Input: part model. Units: mm. Frame: model coordinates. A direction names the side the tool comes from. Round coordinates to 2 decimals unless told otherwise and drop trailing zeros. Loops run counter-clockwise (first coordinate to the right, second up) from the corner with the lowest first, then second, coordinate; pieces in that order, holes last. Notation, with made-up numbers: M 63,-7 L 94,-7 A20 cw 94,2 Z; hole C -24.75,-26 d6. An arc over 180 degrees is marked long. Return JSON: item names as keys, results as strings. Group by question number.
1) Access query for faces 5 (the face through (-66.951, 26, -28)), 6 (the face through (-55, 26, -14)), 7 (the face through (36.8, 56.6, 2.5)), 8 (the face through (-14, 54, 5)), 9 (the face through (-76.951, 29, -27)). Directions: +Z, -Z, +X, -X, +Y, -Y. A direction counts if a zero-diameter tool reaches every point of the face in a straight line with its end or side. Return the directions, or none.
2) Material intervals for line 1 (X direction, y = 29.5, z = -5); line 2 (X direction, y = 34.5, z = -17); line 3 (Z direction, x = 38, y = 52.5), sorted ascending. Write a range as from..to.
3) Mould query, pull axis X, two halves, no side actions, for faces 1 (the face through (7, -9.314, 3)), 2 (the face through (-37.451, 25, -4)), 3 (the face through (80.049, 26, -28)), 4 (the face through (92.049, 28, -30)). Classes: +X half, -X half, draft (parallel to the pull), parting line (faces both ways), or undercut.
4) Section A-A (z = -10). Output: boundary loops of the cut face in (x, y), plus the area to 3 significant figures.
5) Section B-B (x = -52). Output: boundary loops of the cut face in (y, z).
6) Contact query for flat-ended pins moving along their axis: P1, Ø2, axis at x = 63.5, y = 14, coming from the +Z side; P2, Ø5.5, axis at y = 13, z = -29, coming from the -X side; P3, Ø3.5, axis at x = -47.45, y = 55.69, coming from the -Z side; P4, Ø12, axis at x = 52.5, y = 37.5, coming from the -Z side. Output: stop coordinate, or through.
Autodesk Fusion 360 part; units mm, degrees
sketch "Schizzo1" plane through (0, 0, 0) normal (0, 0, 1) x (1, 0, 0)
  line L0 (-32.4508, 65.6855) -> (45.5492, 65.6855)
  line L1 (45.5492, 65.6855) -> (45.5492, -9.3145)
  line L2 (45.5492, -9.3145) -> (-32.4508, -9.3145)
  line L3 (-32.4508, -9.3145) -> (-32.4508, 65.6855)
  line L4 (-32.4508, 28.1855) -> (45.5492, 28.1855) construction
  line L5 (6.5492, 65.6855) -> (6.5492, -9.3145) construction
  circle A0 centre (6.5492, 28.1855) radius 30.5
  line L6 (37.0492, -2.3145) -> (-23.9508, -2.3145) construction
  line L7 (-23.9508, -2.3145) -> (-23.9508, 58.6855) construction
  line L8 (-23.9508, 58.6855) -> (37.0492, 58.6855) construction
  line L9 (37.0492, 58.6855) -> (37.0492, -2.3145) construction
  line L10 (37.0492, -2.3145) -> (-23.9508, 58.6855) construction
  line L11 (-23.9508, -2.3145) -> (37.0492, 58.6855) construction
  circle A1 centre (-23.9508, 58.6855) radius 2.1
  circle A2 centre (37.0492, 58.6855) radius 2.1
  circle A3 centre (37.0492, -2.3145) radius 2.1
  circle A4 centre (-23.9508, -2.3145) radius 2.1
  line L12 (-71.9508, 58.6855) -> (-66.9508, 58.6855)
  line L13 (-66.9508, 58.6855) -> (-66.9508, -2.3145)
  line L14 (-66.9508, -2.3145) -> (-71.9508, -2.3145)
  line L15 (-71.9508, -2.3145) -> (-71.9508, 58.6855)
  line L16 (85.0492, 58.6855) -> (80.0492, 58.6855)
  line L17 (85.0492, -2.3145) -> (85.0492, 58.6855)
  line L18 (80.0492, 58.6855) -> (80.0492, -2.3145)
  line L19 (80.0492, -2.3145) -> (85.0492, -2.3145)
  circle A5 centre (-23.9508, 58.6855) radius 3.6
  circle A6 centre (37.0492, 58.6855) radius 3.6
  circle A7 centre (-23.9508, -2.3145) radius 3.6
  circle A8 centre (37.0492, -2.3145) radius 3.6
  line L20 (-32.4508, -9.3145) -> (-71.9508, -9.3145)
  line L21 (-71.9508, -9.3145) -> (-71.9508, -2.3145)
  line L22 (45.5492, -9.3145) -> (85.0492, -9.3145)
  line L23 (85.0492, -9.3145) -> (85.0492, -2.3145)
  line L24 (-66.9508, -2.3145) -> (-66.9508, -9.3145)
  line L25 (80.0492, -2.3145) -> (80.0492, -9.3145)
  line L26 (-66.9508, 58.6855) -> (-32.4508, 58.6855)
  line L27 (80.0492, 58.6855) -> (45.5492, 58.6855)
  line L28 (-66.9508, 58.6855) -> (-32.4508, 58.6855)
  line L29 (-32.4508, 58.6855) -> (-32.4508, 60.6855)
  line L30 (-32.4508, 60.6855) -> (-66.9508, 60.6855)
  line L31 (-66.9508, 60.6855) -> (-66.9508, 58.6855)
  line L32 (80.0492, 60.6855) -> (80.0492, 58.6855)
  line L33 (45.5492, 60.6855) -> (80.0492, 60.6855)
  line L34 (80.0492, 58.6855) -> (45.5492, 58.6855)
  line L35 (45.5492, -9.3145) -> (45.5492, 65.6855)
  line L36 (-37.4508, -9.3145) -> (-37.4508, 60.6855)
  line L37 (50.5492, -9.3145) -> (50.5492, 60.6855)
  line L38 (-71.9508, 58.6855) -> (-66.9508, 58.6855)
  line L39 (-66.9508, 58.6855) -> (-66.9508, 60.6855)
  line L40 (-66.9508, 60.6855) -> (-71.9508, 60.6855)
  line L41 (-71.9508, 60.6855) -> (-71.9508, 58.6855)
  line L42 (85.0492, 60.6855) -> (85.0492, 58.6855)
  line L43 (80.0492, 60.6855) -> (85.0492, 60.6855)
  point P0 (6.5492, 28.1855)
  point P1 (-23.9508, -2.3145)
  dimension "d1" = 78
  dimension "d2" = 75
  dimension "d3" = 61
  dimension "d4" = 61
  dimension "d5" = 61
  dimension "d6" = 4.2
  dimension "d13" = 5
  dimension "d22" = 7.2
  dimension "d70" = 157
  dimension "d82" = 147
  dimension "d102" = 2
  dimension "d109" = 5
extrude "Estrusione1" add sketch "Schizzo1" along normal blind 5 contours L0 L1 L2 L3 L29 L35 | L3 L26 L28 L29 L30 L36 | L1 L27 L33 L34 L35 L37 | L3 L20 L26 L28 L36 | L1 L22 L27 L34 L35 L37 | A5 | A6 | A7 | A8
fillet "Raccordo22" radius 2 1 edges at (-21.8868, 39.2148, 5)
extrude "Estrusione14" add sketch "Schizzo1" against normal blind 20 contours L3 L26 L28 L29 L30 L36 | L1 L27 L33 L34 L35 L37 | L3 L20 L26 L28 L36 | L1 L22 L27 L34 L35 L37
fillet "Raccordo20" radius 2 2 edges at (-32.4508, 25.6855, 0) (45.5492, 25.6855, 0)
fillet "Raccordo17" radius 2 2 edges at (-32.4508, 65.6855, 2.5) (45.5492, 65.6855, 2.5)
fillet "Raccordo21" radius 2 2 edges at (45.5492, 60.6855, 2.5) (-32.4508, 60.6855, 2.5)
extrude "Estrusione15" add sketch "Schizzo1" along normal blind 6 from surface at -20 contours L3 L20 L26 L28 L36 | L26 L28 L30 L31 L36 L39 | L1 L22 L27 L34 L35 L37 | L27 L32 L33 L34 L37 | L13 L20 L24 L26 L28 L36 | L12 L31 L38 L39 L40 L41 | L18 L22 L25 L27 L34 L37 | L16 L32 L42 L43 | L12 L13 L14 L15 L38 | L16 L17 L18 L19 | L14 L20 L21 L24 | L19 L22 L23 L25
fillet "Raccordo14" radius 2 2 edges at (50.5492, 25.6855, -14) (-37.4508, 25.6855, -14)
fillet "Raccordo18" radius 2 2 edges at (45.5492, 25.6855, -20) (-32.4508, 25.6855, -20)
extrude "Estrusione2" add sketch "Schizzo1" against normal blind 20 from surface at -15 contours L12 L31 L38 L39 L40 L41 | L16 L32 L42 L43 | L12 L13 L14 L15 L38 | L16 L17 L18 L19 | L14 L20 L21 L24 | L19 L22 L23 L25
fillet "Raccordo23" radius 2 2 edges at (-71.9508, 25.6855, -14) (85.0492, 25.6855, -14)
fillet "Raccordo24" radius 2 2 edges at (-66.9508, 25.6855, -20) (80.0492, 25.6855, -20)
sketch "Schizzo2" plane through (-71.9508, 0, 0) normal (-1, 0, 0) x (0, -1, 0)
  line L0 (-60.6855, -35) -> (9.3145, -35)
  circle A0 centre (-28.1855, -30) radius 2.9
  circle A1 centre (-28.1855, -30) radius 3.5
  line L1 (9.3145, -35) -> (9.3145, -16)
  circle A2 centre (0.8145, -30) radius 1.9
  line L2 (-58.6855, -15) -> (9.3145, -15) construction
  line L3 (9.3145, -15) -> (9.3145, -35) construction
  line L4 (9.3145, -35) -> (-58.6855, -35) construction
  line L5 (-58.6855, -35) -> (-58.6855, -15) construction
  line L6 (-58.6855, -30) -> (9.3145, -30) construction
  line L7 (9.3145, -16) -> (-60.6855, -16)
  line L8 (-60.6855, -16) -> (-60.6855, -35)
  dimension "d27" = 5.8
  dimension "d28" = 7
  dimension "d56" = 3.8
  dimension "d94" = 5
  dimension "d95" = 30.5
  dimension "d96" = 29
extrude "Estrusione4" add sketch "Schizzo2" along normal blind 7 contours A0
extrude "Estrusione5" add sketch "Schizzo2" against normal blind 2 from surface at 7 contours A1
fillet "Raccordo4" radius 0.5 1 edges at (-71.9508, 30.8893, -28.9513)
extrude "Estrusione10" cut sketch "Schizzo2" against normal blind 3.5 contours A2
sketch "Schizzo3" plane through (85.0492, 0, 0) normal (1, 0, 0) x (0, 1, 0)
  line L0 (-9.3145, -35) -> (60.6855, -35)
  circle A0 centre (28.1855, -30) radius 2.9
  circle A1 centre (28.1855, -30) radius 3.5
  circle A2 centre (-0.8145, -30) radius 1.9
  line L1 (-9.3145, -16) -> (-9.3145, -35)
  line L2 (58.6855, -35) -> (-9.3145, -35) construction
  line L3 (-9.3145, -35) -> (-9.3145, -15) construction
  line L4 (-9.3145, -15) -> (58.6855, -15) construction
  line L5 (58.6855, -15) -> (58.6855, -35) construction
  line L6 (-9.3145, -30) -> (58.6855, -30) construction
  line L7 (60.6855, -16) -> (-9.3145, -16)
  line L8 (60.6855, -35) -> (60.6855, -16)
  dimension "d36" = 5.8
  dimension "d37" = 7
  dimension "d49" = 3.8
  dimension "d97" = 5
  dimension "d98" = 29
  dimension "d99" = 30.5
extrude "Estrusione6" add sketch "Schizzo3" along normal blind 7 contours A0
extrude "Estrusione7" add sketch "Schizzo3" against normal blind 2 from surface at 7 contours A1
fillet "Raccordo5" radius 0.5 1 edges at (85.0492, 25.4818, -28.9513)
extrude "Estrusione11" cut sketch "Schizzo3" against normal blind 3.5 contours A2
sketch "Schizzo4" plane through (0, 0, 5) normal (0, 0, 1) x (-1, 0, 0)
  line L0 (37.4508, 9.3145) -> (-50.5492, 9.3145)
  line L1 (-43.5492, -65.6855) -> (30.4508, -65.6855)
  circle A0 centre (23.9508, 2.3145) radius 2.1
  circle A1 centre (-37.0492, -58.6855) radius 2.1
  circle A2 centre (23.9508, -58.6855) radius 2.1
  circle A3 centre (-37.0492, 2.3145) radius 2.1
  line L2 (65.9508, -65.6855) -> (-79.0492, -65.6855) construction
  line L3 (-79.0492, -65.6855) -> (-79.0492, 9.3145) construction
  line L4 (-79.0492, 9.3145) -> (65.9508, 9.3145) construction
  line L5 (65.9508, 9.3145) -> (65.9508, -65.6855) construction
  line L6 (-6.5492, -65.6855) -> (-6.5492, 9.3145) construction
  line L7 (-6.5492, -28.1855) -> (65.9508, -28.1855) construction
  line L8 (-6.5492, -28.1855) -> (-79.0492, -28.1855) construction
  line L9 (65.9508, -55.6855) -> (-79.0492, -55.6855) construction
  line L10 (65.9508, -0.6855) -> (-79.0492, -0.6855) construction
  circle A4 centre (47.4508, -55.6855) radius 2.25
  circle A5 centre (47.4508, -55.6855) radius 3.75
  circle A6 centre (51.4508, -0.6855) radius 2.25
  circle A7 centre (51.4508, -0.6855) radius 3.75
  circle A8 centre (-60.5492, -55.6855) radius 2.25
  circle A9 centre (-60.5492, -55.6855) radius 3.75
  circle A10 centre (-64.5492, -0.6855) radius 3.75
  circle A11 centre (-64.5492, -0.6855) radius 2.25
  line L11 (-45.5492, -62.6855) -> (-45.5492, -63.6855)
  line L12 (32.4508, -63.6855) -> (32.4508, -62.6855)
  line L13 (-50.5492, 9.3145) -> (-50.5492, -60.6855)
  line L14 (37.4508, -60.6855) -> (37.4508, 9.3145)
  arc A12 (-45.5492, -63.6855) -> (-43.5492, -65.6855) centre (-43.5492, -63.6855) ccw
  arc A13 (30.4508, -65.6855) -> (32.4508, -63.6855) centre (30.4508, -63.6855) ccw
  circle A14 centre (-6.5492, -28.1855) radius 32.5
  arc A15 (34.4508, -60.6855) -> (32.4508, -62.6855) centre (34.4508, -62.6855) ccw
  line L15 (34.4508, -60.6855) -> (37.4508, -60.6855)
  line L16 (-50.5492, -60.6855) -> (-47.5492, -60.6855)
  arc A16 (-45.5492, -62.6855) -> (-47.5492, -60.6855) centre (-47.5492, -62.6855) ccw
  point P0 (47.4508, -55.6855)
  point P1 (51.4508, -0.6855)
  point P2 (-60.5492, -55.6855)
  point P3 (-64.5492, -0.6855)
  dimension "d79" = 55
  dimension "d80" = 108
  dimension "d81" = 116
  dimension "d83" = 4.5
  dimension "d84" = 7.5
  dimension "d85" = 4.5
  dimension "d86" = 7.5
extrude "Estrusione12" cut sketch "Schizzo4" against normal blind 6 from surface at -19 contours A4 | A6 | A8 | A11
equation "d1 = 75 mm + 0.2 mm + 2.8 mm"
equation "d85 = d83"
equation "d86 = d84"
Returned:
{
 "1": {"face 5": "-Z, +Y, -Y", "face 6": "+Z, -X, +Y, -Y", "face 7": "+Z, -Z", "face 8": "+Z, +X, -X, +Y, -Y", "face 9": "none"},
 "2": {"line 1": "x = -37.45..-32.45, 45.55..50.55", "line 2": "x = -71.95..-32.45, 45.55..85.05", "line 3": "z = 0..5"},
 "3": {"face 1": "draft", "face 2": "-X half", "face 3": "undercut", "face 4": "+X half"},
 "4": {"outline": "M -37.45,-9.31 L -32.45,-9.31 L -32.45,60.69 L -37.45,60.69 Z; M 45.55,-9.31 L 50.55,-9.31 L 50.55,60.69 L 45.55,60.69 Z", "area": "700 mm^2"},
 "5": {"outline": "M -9.31,-20 L -1.5,-20 L -1.5,-14 L -9.31,-14 Z; M 2.87,-20 L 60.69,-20 L 60.69,-14 L 2.87,-14 Z"},
 "6": {"P1": "stops at z = -14", "P2": "stops at x = -71.95", "P3": "passes through", "P4": "stops at z = -20"}
}
